Geometry check sheet. Reference: the model listing, model coordinates, mm. Coordinates: 2 decimals unless noted, no trailing zeros. Order: outer loops, then holes, each group sorted by start corner. A loop starts at its lowest first (then second) coordinate and runs counter-clockwise, first axis right, second up.
Autodesk Inventor part; units mm, degrees
ref_plane "YZ Plane" through (0, 0, 0) normal (1, 0, 0) x (0, 1, 0)
ref_plane "XZ Plane" through (0, 0, 0) normal (0, 1, 0) x (-1, 0, 0)
ref_plane "XY Plane" through (0, 0, 0) normal (0, 0, 1) x (1, 0, 0)
sketch "Sketch2" plane through (0, 0, 0) normal (0, 1, 0) x (-1, 0, 0)
  circle A0 centre (188.3525, 14.1838) radius 2
  circle A1 centre (143.3599, 14.996) radius 2
  circle A2 centre (98.3672, 15.8081) radius 2
  circle A3 centre (53.3745, 16.6203) radius 2
  circle A4 centre (62, 0) radius 2.25
  circle A5 centre (199, 0) radius 2.25
  circle A6 centre (214.5, 0) radius 1.5
  line L0 (217, 7) -> (217, -7)
  line L1 (217, 7) -> (247, 7)
  line L2 (247, 7) -> (247, -7)
  line L3 (217, -7) -> (247, -7)
  circle A7 centre (249.5, 0) radius 1.5
  line L4 (254, 20) -> (254, -20)
  line L5 (254, 20) -> (-23, 25)
  line L6 (-23, 25) -> (-23, -25)
  line L7 (254, -20) -> (-23, -25)
  circle A8 centre (50, -8.5) radius 1.5
  circle A9 centre (-19, -8.5) radius 1.5
  line L8 (45.5, 14.25) -> (45.5, -14.25)
  line L9 (-14.5, -14.25) -> (45.5, -14.25)
  line L10 (-14.5, 14.25) -> (-14.5, -14.25)
  line L11 (-14.5, 14.25) -> (45.5, 14.25)
  circle A10 centre (-19, 8.5) radius 1.5
  circle A11 centre (50, 8.5) radius 1.5
  circle A12 centre (240, 0) radius 1.2295 construction
  circle A13 centre (240, 0) radius 7
  point P0 (0, 0)
  dimension "d77" = 14
  dimension "d28" = 18.5
  dimension "d37" = 20
  dimension "d38" = 20
  dimension "d39" = 42
  dimension "d40" = 21
  dimension "d41" = 50
  dimension "d42" = 10
  dimension "d43" = 10.5
  dimension "d52" = 240
  dimension "d53" = 14
  dimension "d54" = 9.5
  dimension "d62" = 10
  dimension "d73" = 274
  dimension "d74" = 20
extrude "Extrusion2" add sketch "Sketch2" along normal blind 4 contours A0 | A1 | A2 | A3 | A6 | L1 A13 L3 L0 | L1 L2 A13 | A13 L2 L3 | A7 | L4 L7 L6 L5 | A8 | A9 | A10 | A11
properties part number "segment2b" material "Plywood, Finish"
Item 1: Release check for a two-part mould opening along X. For faces 1 (the face through (-246.466, 1.972, 2.681)), 2 (the face through (-114, 4, 0)) record: pulls with the +X half, pulls with the -X half, needs draft (parallel to the pull), parting line crosses it, or undercut.
Item 2: Thickness scan on line 1 along X through (y, z) = (2.75, -7.5); line 2 along X through (y, z) = (1.65, -3.5); line 3 along X through (y, z) = (2.1, -5). Record the ranges inside material, lowest first.
Item 3: Sectioned sample at D-D (x = -80). Record the cut outline in (y, z).
Item 4: Sectioned sample at C-C (x = -240). Record the cut outline in (y, z).
Item 5: Sectioned sample at A-A (x = -32.5). Record the cut outline in (y, z).
Item 6: Sectioned sample at B-B (y = 2.35). Record the cut outline in (x, z), and give its area (3 significant figures).
Item 7: Depth check by flat-ended pin: P1, Ø1.2, axis at x = -0.5, y = 2.5, coming from the +Z side; P2, Ø2, axis at x = -217.5, y = 2.5, coming from the +Z side; P3, Ø1.2, axis at x = -8, y = 1.5, coming from the -Z side; P4, Ø12.5, axis at x = -240, z = 0, coming from the -Y side. Enter the tip coordinate at first touch or a pass-through.
Geometry check:
1. face 1: undercut
1. face 2: needs draft
2. line 1: x = -254 to -45.5, 14.5 to 23
2. line 2: x = -254 to -246.06, -233.94 to -45.5, 14.5 to 23
2. line 3: x = -254 to -244.9, -235.1 to -45.5, 14.5 to 23
3. outline: (0, -23.14) - (4, -23.14) - (4, 23.14) - (0, 23.14) - close
4. outline: (0, -20.25) - (4, -20.25) - (4, -7) - (0, -7) - close; (0, 7) - (4, 7) - (4, 20.25) - (0, 20.25) - close
5. outline: (0, -24) - (4, -24) - (4, -14.25) - (0, -14.25) - close; (0, 14.25) - (4, 14.25) - (4, 24) - (0, 24) - close
6. outline: (-254, -20) - (23, -25) - (23, 25) - (-254, 20) - close; hole circle Ø14 at (-240, 0); hole circle Ø4.5 at (-199, 0); hole circle Ø4.5 at (-62, 0); hole (-45.5, -14.25) - (14.5, -14.25) - (14.5, 14.25) - (-45.5, 14.25) - close
6. area: 10,600 mm2
7. P1: stops at z = 24.59
7. P2: stops at z = 20.68
7. P3: stops at z = -24.45
7. P4: passes through
